Design review of the part shown in the three views and the two pictorial views. Dimensions are in mm from the part's minimum x, y and z. A direction names the side the tool comes from. Round coordinates to 2 decimals unless told otherwise and drop trailing zeros. Order: outer loops, then holes, each group sorted by start corner. A loop starts at its lowest first (then second) coordinate and runs counter-clockwise, first axis right, second up. Notation, with made-up numbers: M 49,-18 L 79,-18 A12 ccw 79,-11 Z; hole C 79.25,-30.5 d5. An arc over 180 degrees is marked long. Use a Markdown table: item, result. Add a question column.
(1) Machinability: for the marked faces 1 and 2, which of the approach directions +Z, -Z, +X, -X, +Y, -Y give a long, thin tool a straight path to every point of the face, cutting with its end or side? Answer none if there is none.
(2) For pin 1 (3 mm diameter, centred on x = 2.5, y = 6, fed in from -Z), flat-tipped, find the tip position at first contact; note if it passes through.
(3) Take a section at C-C (x = 3.75). Write out the cut boundary in (y, z), then the cut area to 3 significant figures.
(4) Take a section at B-B (z = 2.1). Write out the cut boundary in (x, y), then the cut area to 3 significant figures.
(5) Take a section at A-A (y = 3.5). Write out the cut boundary in (x, z).
(6) Take a section at D-D (y = 10). Write out the cut boundary in (x, z), then the cut area to 3 significant figures.
(7) The part is to be moulded in two halves that separate along Z. For the marked faces 3, 4, 5 and 6, say which applies: released by +Z, released by -Z, zero draft, split by the parting line, or undercut.
(8) To check wall thickness, follow probe 1 along Y at (x, z) = (2.75, 1.1); probe 2 along Z at (x, y) = (7.75, 3); probe 3 along Y at (x, z) = (0.75, 0.5). State the ranges of each line that lie inside material, in increasing order. Write a range as from..to.
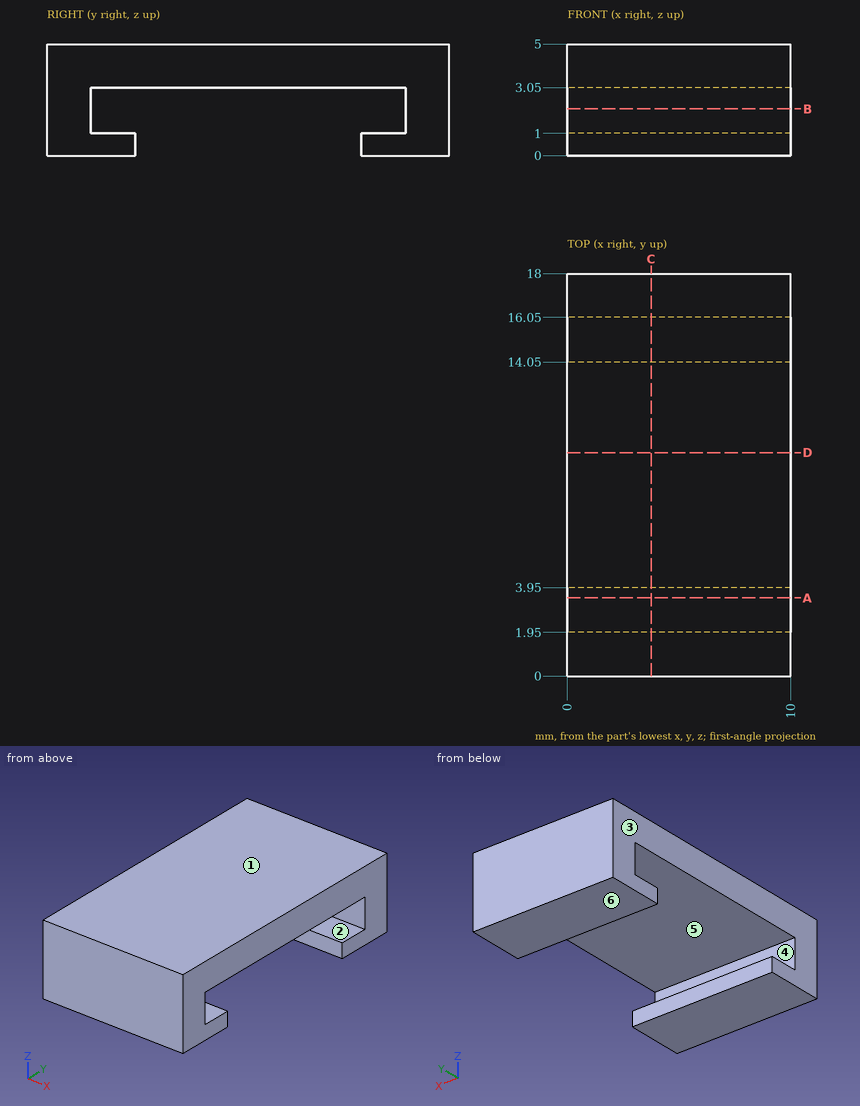
Verdict:
| question | item | result |
|---|---|---|
| 1 | face 1 | +Z, +X, -X, +Y, -Y |
| 1 | face 2 | +X, -X |
| 2 | pin 1 | stops at z = 3.05 |
| 3 | outline | M 0,0 L 3.95,0 L 3.95,1 L 1.95,1 L 1.95,3.05 L 16.05,3.05 L 16.05,1 L 14.05,1 L 14.05,0 L 18,0 L 18,5 L 0,5 Z |
| 3 | area | 51.0 mm^2 |
| 4 | outline | M 0,0 L 10,0 L 10,1.95 L 0,1.95 Z; M 0,16.05 L 10,16.05 L 10,18 L 0,18 Z |
| 4 | area | 39.0 mm^2 |
| 5 | outline | M 0,0 L 10,0 L 10,1 L 0,1 Z; M 0,3.05 L 10,3.05 L 10,5 L 0,5 Z |
| 6 | outline | M 0,3.05 L 10,3.05 L 10,5 L 0,5 Z |
| 6 | area | 19.5 mm^2 |
| 7 | face 3 | zero draft |
| 7 | face 4 | undercut |
| 7 | face 5 | undercut |
| 7 | face 6 | released by -Z |
| 8 | probe 1 | y = 0..1.95, 16.05..18 |
| 8 | probe 2 | z = 0..1, 3.05..5 |
| 8 | probe 3 | y = 0..3.95, 14.05..18 |
